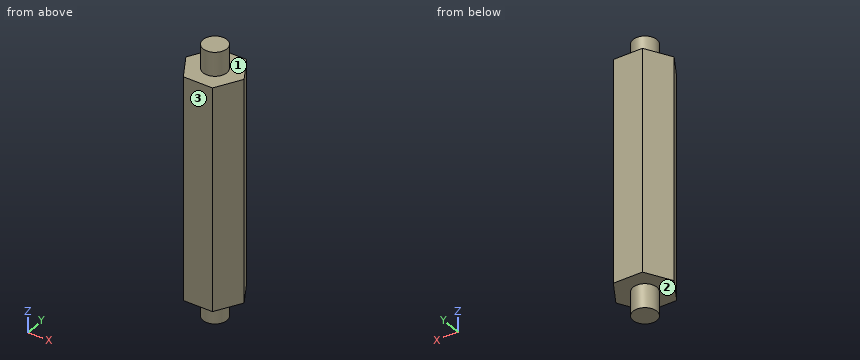
from build123d import *

# Parameters (mm, degrees)
F0_R     = 1.5
F1_DEPTH = 3
F2_R     = 1.5
F3_DEPTH = 28
F4_R     = 1.5
F5_DEPTH = 3


with BuildPart() as f1:
    # F0 (on Top) → F1 (new body)
    with BuildSketch(Plane.XY):
        Circle(F0_R)
    extrude(amount=F1_DEPTH)

    # F2 (on face) → F3 (join)
    with BuildSketch(Plane.XY.offset(3)):
        Polygon((1.8186533479, 3.15), (-1.8186533479, 3.15), (-3.6373066959, 0), (-1.8186533479, -3.15), (1.8186533479, -3.15), (3.6373066959, 0), align=None)
        Circle(F2_R, mode=Mode.SUBTRACT)
        Circle(F2_R)
    extrude(amount=F3_DEPTH)

    # F4 (on face) → F5 (join)
    with BuildSketch(Plane.XY.offset(31)):
        Circle(F4_R)
    extrude(amount=F5_DEPTH)


solid = f1.part
Check sheet for the modelled part. Datum: model origin and axes. Units: mm. Face numbers are marked on the shaded views. A direction names the side the tool comes from. Give positions to 0.01 mm unless a question says otherwise; leave off trailing zeros. Write each loop counter-clockwise with the first axis right and the second up, starting at its lowest first coordinate (ties: lowest second). Pieces come first, ordered by that corner, then holes. Notation, with made-up numbers: (-8, 37) -> (35, 37) arc R25 cw to (35, 60) -> close; hole circle Ø10 at (81, 41). An arc over 180 degrees is marked (long way). One line per item, written item: value. Start each with the question number.
Item 1: Section check D-D on z = 32. Record the cut outline in (x, y).
Item 2: Section check C-C on y = -0.5. Record the cut outline in (x, z), then the cut area to 3 significant figures.
Item 3: Tool access check on the marked faces 1, 2 and 3. Record the directions out of +Z, -Z, +X, -X, +Y, -Y that give a thin tool (end or side, any length) a straight path to the whole face; none if there is none.
Item 4: Section check B-B on x = 0. Record the cut outline in (y, z).
Item 5: Material ranges on probe 1 along Z at (x, y) = (-1.25, -1); probe 2 along Y at (x, z) = (-2.25, 8); probe 3 along X at (y, z) = (-1.25, 27), recorded low to high. Write a range as from..to.
Item 6: Section check A-A on z = 8. Record the cut outline in (x, y).
Results list:
1. outline: circle Ø3 at (0, 0)
2. outline: (-3.35, 3) -> (-1.41, 3) -> (-1.41, 0) -> (1.41, 0) -> (1.41, 3) -> (3.35, 3) -> (3.35, 31) -> (1.41, 31) -> (1.41, 34) -> (-1.41, 34) -> (-1.41, 31) -> (-3.35, 31) -> close
2. area: 204 mm²
3. face 1: +Z
3. face 2: -Z
3. face 3: +Z, -Z, +X, -X, -Y
4. outline: (-3.15, 3) -> (-1.5, 3) -> (-1.5, 0) -> (1.5, 0) -> (1.5, 3) -> (3.15, 3) -> (3.15, 31) -> (1.5, 31) -> (1.5, 34) -> (-1.5, 34) -> (-1.5, 31) -> (-3.15, 31) -> close
5. probe 1: 3..31
5. probe 2: -2.4..2.4
5. probe 3: -2.92..2.92
6. outline: (-3.64, 0) -> (-1.82, -3.15) -> (1.82, -3.15) -> (3.64, 0) -> (1.82, 3.15) -> (-1.82, 3.15) -> close
